from build123d import *

# Parameters (mm, degrees)
EXTRUDE_1_OUTLINE_W   = 10
EXTRUDE_1_OUTLINE_H   = 10
EXTRUDE_1_OUTLINE_W_2 = 8
EXTRUDE_1_OUTLINE_H_2 = 8
EXTRUDE_1_DEPTH       = 400
SKETCH_2_R            = 1.6
CUT_EXTRUDE_1_DEPTH   = 401.156219494
SKETCH_3_R            = 1.6
CUT_EXTRUDE_2_DEPTH   = 401.156219494


# Read off the part's stored shape, not the designer's step: 押し出し-薄板1
with BuildPart() as part:
    # 押し出し-薄板1 outline → 押し出し-薄板1 (new body)
    with BuildSketch(Plane.XY):
        Rectangle(EXTRUDE_1_OUTLINE_W, EXTRUDE_1_OUTLINE_H)
        Rectangle(EXTRUDE_1_OUTLINE_W_2, EXTRUDE_1_OUTLINE_H_2, mode=Mode.SUBTRACT)
    extrude(amount=EXTRUDE_1_DEPTH)

    # ｽｹｯﾁ2 → ｶｯﾄ - 押し出し1 (cut, through all)
    with BuildSketch(Plane(origin=(0, 5, 0), x_dir=(1, 0, 0), z_dir=(0, 1, 0))):
        with Locations(Location((0, -355, 0), (0, 0, 270))):
            Circle(SKETCH_2_R)
        with Locations(Location((0, -45, 0), (0, 0, 270))):
            Circle(SKETCH_2_R)
        with Locations(Location((0, -305, 0), (0, 0, 270))):
            Circle(SKETCH_2_R)
        with Locations(Location((0, -95, 0), (0, 0, 270))):
            Circle(SKETCH_2_R)
        with Locations(Location((0, -395, 0), (0, 0, 270))):
            Circle(SKETCH_2_R)
        with Locations(Location((0, -5, 0), (0, 0, 270))):
            Circle(SKETCH_2_R)
    extrude(amount=-CUT_EXTRUDE_1_DEPTH, mode=Mode.SUBTRACT)

    # ｽｹｯﾁ3 → ｶｯﾄ - 押し出し2 (cut, through all)
    with BuildSketch(Plane(origin=(5, 0, 0), x_dir=(0, 0, -1), z_dir=(1, 0, 0))):
        with Locations((-385, 0)):
            Circle(SKETCH_3_R)
        with Locations((-15, 0)):
            Circle(SKETCH_3_R)
    extrude(amount=-CUT_EXTRUDE_2_DEPTH, mode=Mode.SUBTRACT)


solid = part.part
Can you work these out from the model? Positions are in its coordinate system, mm. A direction names the side the tool comes from. Round coordinates to 2 decimals unless told otherwise and drop trailing zeros. Loops run counter-clockwise (first coordinate to the right, second up) from the corner with the lowest first, then second, coordinate; pieces in that order, holes last. Notation, with made-up numbers: (-30.75, 0.5) - (2.25, 0.5) arc R17 cw to (2.25, 12.5) - close; hole circle Ø3 at (-12.75, -2.5). An arc over 180 degrees is marked (long way). Answer in a Markdown table with one row per item. Add a question column.
Q1. I want a section at A-A on z = 217.5. List the corners of the cut face in (x, y) for me, and give its area (3 significant figures).
Q2. For pin 1 Ø1.9 at (x, z) = (0, 45) entering from -Y, with a flat end and sliding along its axis, tell me the tip position at first contact or that it passes through.
Q3. We'd pull the mould along X, two halves only. Please class faces 1 (the flat face through (0, 4, 197)), 2 (the flat face through (-5, 0, 197)), 3 (the flat face through (0, -5, 197)), 4 (the flat face through (0, -4, 197)): pulls with the +X half, pulls with the -X half, needs draft (parallel to the pull), parting line crosses it, or undercut.
Q4. I want a section at B-B on x = 0. Count the separate pieces of the cut face and the enclosed holes in it, and give its area (3 significant figures).
Q5. I need wall thicknesses on L1, parallel to Y at x = -3, z = 222; L2, parallel to X at y = -4.7, z = 5. Which ranges of each line are inside material? Lowest first, please.
Q6. Which directions (+Z, -Z, +X, -X, +Y, -Y) give clear straight access to the entire face, cutting with the end or side of a thin tool? Please do faces 5 (the flat face through (4, 0, 197)), 6 (the flat face through (-4.5, 0.1, 400)).
A:
| question | item | result |
|---|---|---|
| 1 | outline | (-5, -5) - (5, -5) - (5, 5) - (-5, 5) - close; hole (-4, -4) - (4, -4) - (4, 4) - (-4, 4) - close |
| 1 | area | 36.0 mm^2 |
| 2 | pin 1 | through |
| 3 | face 1 | undercut |
| 3 | face 2 | pulls with the -X half |
| 3 | face 3 | needs draft |
| 3 | face 4 | undercut |
| 4 | separate pieces | 14 |
| 4 | enclosed holes | 0 |
| 4 | area | 762 mm^2 |
| 5 | L1 | -5 to -4, 4 to 5 |
| 5 | L2 | -5 to -1.6, 1.6 to 5 |
| 6 | face 5 | +Z, -Z |
| 6 | face 6 | +Z, +X, -X, +Y, -Y |
